Check sheet for the modelled part. Datum: model origin and axes. Units: mm. Face numbers are marked on the shaded views. A direction names the side the tool comes from. Round coordinates to 2 decimals unless told otherwise and drop trailing zeros. Write each loop counter-clockwise with the first axis right and the second up, starting at its lowest first coordinate (ties: lowest second). Pieces come first, ordered by that corner, then holes. Notation, with made-up numbers: M 64,-12 L 96,-12 A22 cw 96,10 Z; hole C 81.25,3 d11. An arc over 180 degrees is marked long. Put each result on its own line as item: value.
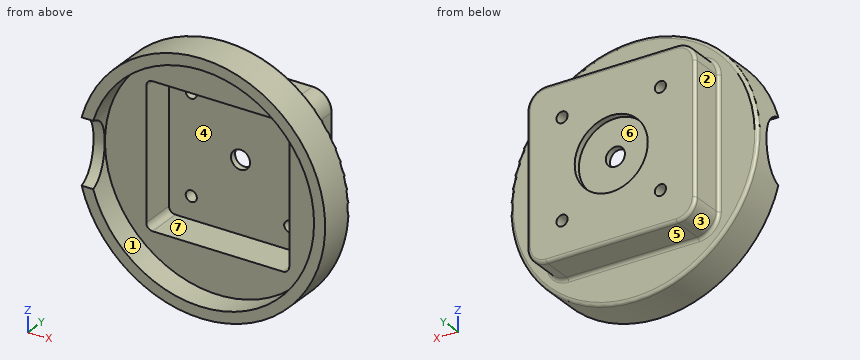
```python
from build123d import *

# Parameters (mm, degrees)
SKETCH1_R           = 39
SKETCH1_R_2         = 35.5
BOSS_EXTRUDE1_DEPTH = 8
SKETCH2_R           = 39
BOSS_EXTRUDE2_DEPTH = 4
BOSS_EXTRUDE3_DEPTH = 7
BOSS_EXTRUDE4_DEPTH = 4
SKETCH5_R           = 11.5
CUT_EXTRUDE1_DEPTH  = 2
SKETCH6_R           = 1.75
SKETCH6_R_2         = 3
CUT_EXTRUDE2_DEPTH  = 60.757844673
FILLET1_R           = 1
FILLET2_R           = 1
SKETCH7_R           = 10.6
CUT_EXTRUDE3_DEPTH  = 50


with BuildPart() as part:
    # Sketch1 → Boss-Extrude1 (new body)
    with BuildSketch(Plane(origin=(0, 0, 0), x_dir=(1, 0, 0), z_dir=(0, 1, 0))):
        with Locations(Location((0, 0, 0), (0, 0, 270))):
            Circle(SKETCH1_R)
        with Locations(Location((0, 0, 0), (0, 0, 270))):
            Circle(SKETCH1_R_2, mode=Mode.SUBTRACT)
    extrude(amount=BOSS_EXTRUDE1_DEPTH)

    # Sketch2 → Boss-Extrude2 (add)
    with BuildSketch(Plane(origin=(0, 8, 0), x_dir=(1, 0, 0), z_dir=(0, 1, 0))):
        with Locations(Location((0, 0, 0), (0, 0, 270))):
            Circle(SKETCH2_R)
        with BuildLine():
            Line((-20.5, -22.5), (20.5, -22.5))
            ThreePointArc((20.5, -22.5), (21.914213562, -21.914213562), (22.5, -20.5))
            Line((22.5, -20.5), (22.5, 20.5))
            ThreePointArc((22.5, 20.5), (21.914213562, 21.914213562), (20.5, 22.5))
            Line((20.5, 22.5), (-20.5, 22.5))
            ThreePointArc((-20.5, 22.5), (-21.914213562, 21.914213562), (-22.5, 20.5))
            Line((-22.5, 20.5), (-22.5, -20.5))
            ThreePointArc((-22.5, -20.5), (-21.914213562, -21.914213562), (-20.5, -22.5))
        make_face(mode=Mode.SUBTRACT)
    extrude(amount=BOSS_EXTRUDE2_DEPTH)

    # Sketch3 → Boss-Extrude3 (add)
    with BuildSketch(Plane(origin=(0, 12, 0), x_dir=(1, 0, 0), z_dir=(0, 1, 0))):
        with BuildLine():
            Line((-20.5, -26.5), (20.5, -26.5))
            ThreePointArc((20.5, -26.5), (24.742640687, -24.742640687), (26.5, -20.5))
            Line((26.5, -20.5), (26.5, 20.5))
            ThreePointArc((26.5, 20.5), (24.742640687, 24.742640687), (20.5, 26.5))
            Line((20.5, 26.5), (-20.5, 26.5))
            ThreePointArc((-20.5, 26.5), (-24.742640687, 24.742640687), (-26.5, 20.5))
            Line((-26.5, 20.5), (-26.5, -20.5))
            ThreePointArc((-26.5, -20.5), (-24.742640687, -24.742640687), (-20.5, -26.5))
        make_face()
        with BuildLine():
            Line((-20.5, -22.5), (20.5, -22.5))
            ThreePointArc((20.5, -22.5), (21.914213562, -21.914213562), (22.5, -20.5))
            Line((22.5, -20.5), (22.5, 20.5))
            ThreePointArc((22.5, 20.5), (21.914213562, 21.914213562), (20.5, 22.5))
            Line((20.5, 22.5), (-20.5, 22.5))
            ThreePointArc((-20.5, 22.5), (-21.914213562, 21.914213562), (-22.5, 20.5))
            Line((-22.5, 20.5), (-22.5, -20.5))
            ThreePointArc((-22.5, -20.5), (-21.914213562, -21.914213562), (-20.5, -22.5))
        make_face(mode=Mode.SUBTRACT)
    extrude(amount=BOSS_EXTRUDE3_DEPTH)

    # Sketch4 → Boss-Extrude4 (add)
    with BuildSketch(Plane(origin=(0, 19, 0), x_dir=(1, 0, 0), z_dir=(0, 1, 0))):
        with BuildLine():
            Line((-20.5, -26.5), (20.5, -26.5))
            ThreePointArc((20.5, -26.5), (24.742640687, -24.742640687), (26.5, -20.5))
            Line((26.5, -20.5), (26.5, 20.5))
            ThreePointArc((26.5, 20.5), (24.742640687, 24.742640687), (20.5, 26.5))
            Line((20.5, 26.5), (-20.5, 26.5))
            ThreePointArc((-20.5, 26.5), (-24.742640687, 24.742640687), (-26.5, 20.5))
            Line((-26.5, 20.5), (-26.5, -20.5))
            ThreePointArc((-26.5, -20.5), (-24.742640687, -24.742640687), (-20.5, -26.5))
        make_face()
    extrude(amount=BOSS_EXTRUDE4_DEPTH)

    # Sketch5 → Cut-Extrude1 (cut)
    with BuildSketch(Plane(origin=(0, 23, 0), x_dir=(1, 0, 0), z_dir=(0, 1, 0))):
        with Locations(Location((0, 0, 0), (0, 0, 270))):
            Circle(SKETCH5_R)
    extrude(amount=-CUT_EXTRUDE1_DEPTH, mode=Mode.SUBTRACT)

    # Sketch6 → Cut-Extrude2 (cut, through all)
    with BuildSketch(Plane(origin=(0, 23, 0), x_dir=(1, 0, 0), z_dir=(0, 1, 0))):
        with Locations(Location((-15.485638508, 15.485638508, 0), (0, 0, 270))):
            Circle(SKETCH6_R)
        with Locations(Location((15.485638508, 15.485638508, 0), (0, 0, 270))):
            Circle(SKETCH6_R)
        with Locations(Location((15.485638508, -15.485638508, 0), (0, 0, 270))):
            Circle(SKETCH6_R)
        with Locations(Location((-15.485638508, -15.485638508, 0), (0, 0, 270))):
            Circle(SKETCH6_R)
        with Locations(Location((0, 0, 0), (0, 0, 270))):
            Circle(SKETCH6_R_2)
    extrude(amount=-CUT_EXTRUDE2_DEPTH, mode=Mode.SUBTRACT)

    # Fillet1
    fillet1_edges = [part.edges().sort_by_distance(p)[0] for p in [
        (-24.742640687, 12, 24.742640687),
        (0, 12, 26.5),
        (24.742640687, 12, 24.742640687),
        (26.5, 12, 0),
        (24.742640687, 12, -24.742640687),
        (0, 12, -26.5),
        (-24.742640687, 12, -24.742640687),
        (-26.5, 12, 0),
        (0, 12, -39),
    ]]
    fillet(fillet1_edges, radius=FILLET1_R)

    # Fillet2
    fillet2_edges = [part.edges().sort_by_distance(p)[0] for p in [
        (-24.742640687, 23, 24.742640687),
        (0, 23, 26.5),
        (24.742640687, 23, 24.742640687),
        (26.5, 23, 0),
        (24.742640687, 23, -24.742640687),
        (0, 23, -26.5),
        (-24.742640687, 23, -24.742640687),
        (-26.5, 23, 0),
    ]]
    fillet(fillet2_edges, radius=FILLET2_R)

    # Sketch7 → Cut-Extrude3 (cut)
    with BuildSketch(Plane(origin=(0, 0, 0), x_dir=(0, 0, -1), z_dir=(1, 0, 0))):
        with Locations((0, -2.75)):
            Circle(SKETCH7_R)
    extrude(amount=-CUT_EXTRUDE3_DEPTH, mode=Mode.SUBTRACT)


solid = part.part
```
1. Cross-section at C-C (y = 2). Enter the section's corners in (x, z), then the cut area to 3 significant figures.
Computed values:
outline: M -37.83,-9.48 A39 ccw long -37.83,9.48 L -34.21,9.48 A35.5 cw long -34.21,-9.48 Z
area: 752 mm2
2. Access from +Z, -Z, +X, -X, +Y, -Y to the whole of each face (thin tool, end or side, straight path). Record for the marked faces 5, 6 and 7.
Computed values:
face 5: -Z, +X, -X, +Y
face 6: +Y
face 7: -Y
3. Scan lines: probe 1 along Z at (x, y) = (0, 6.5); probe 2 along Z at (x, y) = (-1, 11); probe 3 along X at (y, z) = (13.5, 13.5). Record each from-to range of solid material in increasing order.
Computed values:
probe 1: z = -39 to -35.5, 35.5 to 39
probe 2: z = -38.99 to -22.5, 22.5 to 38.99
probe 3: x = -26.5 to -22.5, 22.5 to 26.5
4. Release check for a two-part mould opening along Z. For the marked faces 1, 2, 3 and 4 record: +Z half, -Z half, draft (parallel to the pull), parting line (faces both ways), or undercut.
Computed values:
face 1: undercut
face 2: draft
face 3: -Z half
face 4: undercut
5. Depth check by flat-ended pin: pin 1 Ø1 at (x, y) = (-12.5, 19) entering from +Z; pin 2 Ø3 at (y, z) = (19, -1.5) entering from -X; pin 3 Ø4.5 at (y, z) = (16, -8) entering from +X; pin 4 Ø3 at (x, z) = (-15.49, -15.49) entering from -Y. Enter the tip coordinate at first touch or a pass-through.
Computed values:
pin 1: stops at z = 26.5
pin 2: stops at x = -26.5
pin 3: stops at x = 26.5
pin 4: passes through
